from build123d import *

# Parameters (mm, degrees)
BOSS_EXTRUDE1_DEPTH = 6.5
M8_TAPPED_HOLE1_D   = 6.8
CHAMFER1_SIZE       = 1


with BuildPart() as part:
    # Sketch1 → Boss-Extrude1 (new body)
    with BuildSketch(Plane(origin=(0, 0, 0), x_dir=(1, 0, 0), z_dir=(0, 1, 0))):
        Polygon((3.75277675, 6.5), (-3.75277675, 6.5), (-7.505553499, 0), (-3.75277675, -6.5), (3.75277675, -6.5), (7.505553499, 0), align=None)
    extrude(amount=BOSS_EXTRUDE1_DEPTH)

    # Sketch2 → Cut-Revolve1 (revolve, cut)
    with BuildSketch(Plane(origin=(0, 0, 0), x_dir=(0, 0, -1), z_dir=(1, 0, 0))):
        Polygon((-9.964101615, 6.5), (-9.964101615, 4.5), (-6.5, 6.5), align=None)
        Polygon((-9.964101615, 2), (-6.5, 0), (-9.964101615, 0), align=None)
    revolve(axis=Axis((0, 0, 0), (0, 1, 0)), mode=Mode.SUBTRACT)

    # M8 Tapped Hole1 (through all)
    with Locations(Plane(origin=(0, 6.5, 0), x_dir=(-1, 0, 0), z_dir=(0, 1, 0))):
        with Locations((0, 0)):
            Hole(M8_TAPPED_HOLE1_D / 2)

    # Chamfer1
    chamfer1_edges = [part.edges().sort_by_distance(p)[0] for p in [
        (-3.4, 6.5, 0),
        (-3.4, 0, 0),
    ]]
    chamfer(chamfer1_edges, length=CHAMFER1_SIZE)


solid = part.part
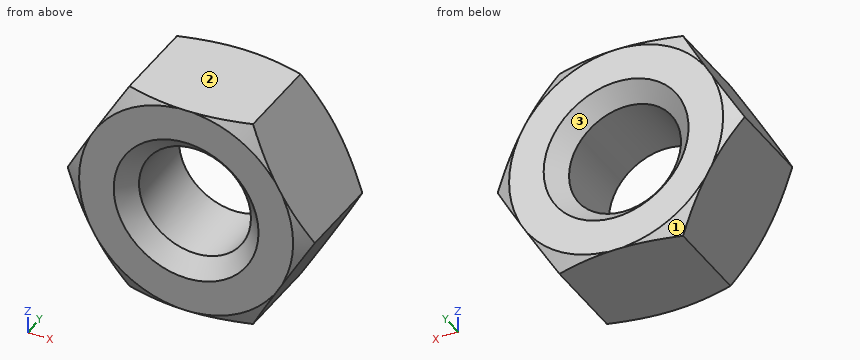
The listing builds one solid part. Answer for the finished solid, in the listing's coordinates (mm). Face numbers are marked on the shaded views. Round coordinates to 2 decimals unless told otherwise and drop trailing zeros. Loops run counter-clockwise (first coordinate to the right, second up) from the corner with the lowest first, then second, coordinate; pieces in that order, holes last. Notation, with made-up numbers: M -4.75,15 L 18.25,15 A19 cw 18.25,40 Z; hole C -3.75,5 d4. An arc over 180 degrees is marked long. Write each question's results on one line, items separated by ' | '. Start each with the question number.
1) This flat-tipped pin is pushed along its axis until it touches: pin 1 (1.5 mm diameter, centred on y = 3.5, z = -4.5, fed in from -X). Where does it stop, or does it pass through?
2) Find section A-A on y = 2.5. Write down the section's boundary in (x, z), plus the area to 3 significant figures.
3) Straight lines are drawn through the part: probe 1 along Z at (x, y) = (0, 3.35); probe 2 along Z at (x, y) = (-2, 5.25); probe 3 along X at (y, z) = (0.5, 2). For each, find the intervals that lie inside material, in ascending order.
4) Determine the mould class of the marked faces 1, 2 and 3 for opening direction Z: pulls with the +Z half, pulls with the -Z half, needs draft (parallel to the pull), parting line crosses it, or undercut.
Final values:
1) pin 1: x = -5.34
2) outline: M -7.51,0 L -3.75,-6.5 L 3.75,-6.5 L 7.51,0 L 3.75,6.5 L -3.75,6.5 Z; hole C 0,0 d6.8 | area: 110 mm²
3) probe 1: -6.5 to -3.4, 3.4 to 6.5 | probe 2: -6.5 to -2.75, 2.75 to 6.5 | probe 3: -6.35 to -3.35, 3.35 to 6.35
4) face 1: pulls with the -Z half | face 2: pulls with the +Z half | face 3: undercut
